Geometry check sheet. Reference: the model listing, model coordinates, mm. Face numbers are marked on the shaded views. A direction names the side the tool comes from. Coordinates: 2 decimals unless noted, no trailing zeros. Order: outer loops, then holes, each group sorted by start corner. A loop starts at its lowest first (then second) coordinate and runs counter-clockwise, first axis right, second up. Notation, with made-up numbers: (-31, 42) - (22, 42) arc R26 cw to (22, 62) - close; hole circle Ø6 at (30, -27.75). An arc over 180 degrees is marked (long way). Return JSON: item names as keys, results as strings. Group by question number.
Item 1: Section check B-B on x = 0. Enter the section's corners in (y, z), then the cut area to 3 significant figures.
Item 2: Tool access check on the marked faces 1, 2 and 3. Record the directions out of +Z, -Z, +X, -X, +Y, -Y that give a thin tool (end or side, any length) a straight path to the whole face; none if there is none.
Item 3: Scan lines: probe 1 along Y at (x, z) = (0, 14); probe 2 along Y at (x, z) = (-2, 13.5); probe 3 along Z at (x, y) = (-22, 4.5). Record each from-to range of solid material in increasing order.
Item 4: Gauge pin test, flat ends, axial feed: pin 1 (2 mm diameter, centred on y = 29, z = 22.5, fed in from +X); pin 2 (3.5 mm diameter, centred on x = -44.5, z = 27.5, fed in from +Y); pin 3 (11.5 mm diameter, centred on x = 0, y = 0, fed in from -Z); pin 4 (2 mm diameter, centred on x = -12.5, z = 10.5, fed in from +Y). Record the tip position at first contact, or that the pin passes through.
Item 5: Section check C-C on y = 3.5. Enter the section's corners in (x, z), then the cut area to 3 significant figures.
Item 6: Section check D-D on x = -43.5. Enter the section's corners in (y, z).
Item 7: Draft check along X on the marked faces 4, 5 and 6. Enter one of: pulls with the +X half, pulls with the -X half, needs draft (parallel to the pull), parting line crosses it, or undercut.
Item 8: Section check A-A on z = 22. Enter the section's corners in (x, y).
from build123d import *

# Parameters (mm, degrees)
SKETCH1_R           = 60
BOSS_EXTRUDE1_DEPTH = 32
CUT_EXTRUDE1_DEPTH  = 12
CUT_EXTRUDE2_DEPTH  = 12
SKETCH4_R           = 5
CUT_EXTRUDE3_DEPTH  = 92


with BuildPart() as part:
    # Sketch1 → Boss-Extrude1 (new body)
    with BuildSketch(Plane.XY):
        Circle(SKETCH1_R)
    extrude(amount=BOSS_EXTRUDE1_DEPTH)

    # Sketch2 → Cut-Extrude1 (cut)
    with BuildSketch(Plane.XY.offset(32)):
        with BuildLine():
            Line((12, -12), (72.488491821, -12))
            Line((72.488491821, -12), (72.488491821, 12))
            Line((72.488491821, 12), (12, 12))
            Line((12, 12), (12, 25))
            ThreePointArc((12, 25), (0, 37), (-12, 25))
            Line((-12, 25), (-12, 12))
            Line((-12, 12), (-72.488491821, 12))
            Line((-72.488491821, 12), (-72.488491821, -12))
            Line((-72.488491821, -12), (-12, -12))
            Line((-12, -12), (-12, -25))
            ThreePointArc((-12, -25), (0, -37), (12, -25))
            Line((12, -25), (12, -12))
        make_face()
    extrude(amount=-CUT_EXTRUDE1_DEPTH, mode=Mode.SUBTRACT)

    # Sketch3 → Cut-Extrude2 (cut)
    with BuildSketch(Plane.XY.offset(32)):
        with BuildLine():
            ThreePointArc((21.5, -37.239092363), (29.696152423, -39.435244785), (27.5, -47.631397208))
            ThreePointArc((27.5, -47.631397208), (0, -55), (-27.5, -47.631397208))
            ThreePointArc((-27.5, -47.631397208), (-29.696152423, -39.435244785), (-21.5, -37.239092363))
            ThreePointArc((-21.5, -37.239092363), (0, -43), (21.5, -37.239092363))
        make_face()
        with BuildLine():
            ThreePointArc((27.5, 47.631397208), (0, 55), (-27.5, 47.631397208))
            ThreePointArc((-27.5, 47.631397208), (-29.696152423, 39.435244785), (-21.5, 37.239092363))
            ThreePointArc((-21.5, 37.239092363), (0, 43), (21.5, 37.239092363))
            ThreePointArc((21.5, 37.239092363), (29.696152423, 39.435244785), (27.5, 47.631397208))
        make_face()
    extrude(amount=-CUT_EXTRUDE2_DEPTH, mode=Mode.SUBTRACT)

    # Sketch4 → Cut-Extrude3 (cut)
    with BuildSketch(Plane.XY.offset(20)):
        Circle(SKETCH4_R)
        with Locations((40, 0)):
            Circle(SKETCH4_R)
        with Locations((0, 30)):
            Circle(SKETCH4_R)
        with Locations((0, -30)):
            Circle(SKETCH4_R)
        with Locations((-40, 0)):
            Circle(SKETCH4_R)
    extrude(amount=-CUT_EXTRUDE3_DEPTH, mode=Mode.SUBTRACT)


solid = part.part
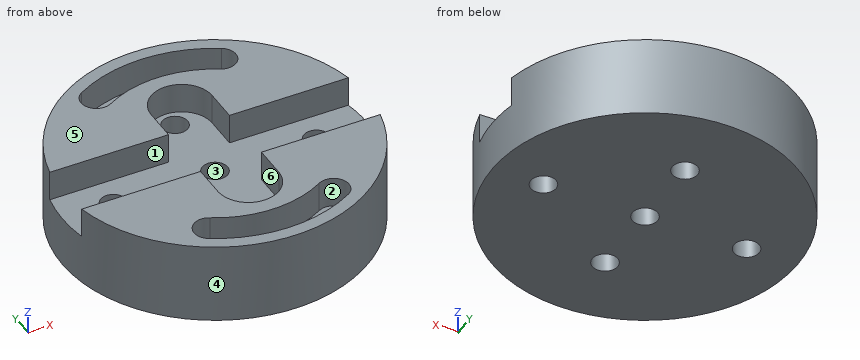
Computed:
{
 "1": {"outline": "(-60, 0) - (-35, 0) - (-35, 20) - (-37, 20) - (-37, 32) - (-43, 32) - (-43, 20) - (-55, 20) - (-55, 32) - (-60, 32) - close; (-25, 0) - (-5, 0) - (-5, 20) - (-25, 20) - close; (5, 0) - (25, 0) - (25, 20) - (5, 20) - close; (35, 0) - (60, 0) - (60, 32) - (55, 32) - (55, 20) - (43, 20) - (43, 32) - (37, 32) - (37, 20) - (35, 20) - close", "area": "2,060 mm²"},
 "2": {"face 1": "+Z, +X, -X", "face 2": "+Z", "face 3": "+Z, -Z"},
 "3": {"probe 1": "y = -60 to -35, -25 to -5, 5 to 25, 35 to 60", "probe 2": "y = -59.97 to -34.58, -25.42 to -4.58, 4.58 to 25.42, 34.58 to 59.97", "probe 3": "z = 0 to 20"},
 "4": {"pin 1": "stops at x = 53.07", "pin 2": "stops at y = 42.1", "pin 3": "stops at z = 0", "pin 4": "stops at y = 58.89"},
 "5": {"outline": "(-59.9, 0) - (-43.57, 0) - (-43.57, 20) - (-59.9, 20) - close; (-36.43, 0) - (-3.57, 0) - (-3.57, 20) - (-36.43, 20) - close; (3.57, 0) - (36.43, 0) - (36.43, 20) - (3.57, 20) - close; (43.57, 0) - (59.9, 0) - (59.9, 20) - (43.57, 20) - close", "area": "1,970 mm²"},
 "6": {"outline": "(-41.32, 0) - (-3.57, 0) - (-3.57, 20) - (-12, 20) - (-12, 32) - (-41.32, 32) - close; (3.57, 0) - (41.32, 0) - (41.32, 32) - (12, 32) - (12, 20) - (3.57, 20) - close"},
 "7": {"face 4": "parting line crosses it", "face 5": "needs draft", "face 6": "undercut"},
 "8": {"outline": "(-58.79, -12) arc R60 ccw to (58.79, -12) - (12, -12) - (12, -25) arc R12 cw to (-12, -25) - (-12, -12) - close; (-58.79, 12) - (-12, 12) - (-12, 25) arc R12 cw to (12, 25) - (12, 12) - (58.79, 12) arc R60 ccw to start; hole (-27.5, -47.63) arc R55 ccw to (27.5, -47.63) arc R6 ccw to (21.5, -37.24) arc R43 cw to (-21.5, -37.24) arc R6 ccw to start; hole (-27.5, 47.63) arc R6 ccw to (-21.5, 37.24) arc R43 cw to (21.5, 37.24) arc R6 ccw to (27.5, 47.63) arc R55 ccw to start"}
}
